```python
from build123d import *

# Parameters (mm, degrees)
SKETCH1_W           = 150
SKETCH1_H           = 150
BOSS_EXTRUDE1_DEPTH = 3
SKETCH2_R           = 2.125
SKETCH2_R_2         = 25
CUT_EXTRUDE3_DEPTH  = 107.108435103
SKETCH3_W           = 10
SKETCH3_H           = 74
SKETCH3_R           = 2.125
BOSS_EXTRUDE2_DEPTH = 3
BOSS_EXTRUDE3_DEPTH = 3


with BuildPart() as part:
    # Sketch1 → Boss-Extrude1 (new body)
    with BuildSketch(Plane(origin=(0, 0, 0), x_dir=(1, 0, 0), z_dir=(0, 1, 0))):
        Rectangle(SKETCH1_W, SKETCH1_H)
    extrude(amount=BOSS_EXTRUDE1_DEPTH)

    # Sketch2 → Cut-Extrude3 (cut, through all)
    with BuildSketch(Plane(origin=(0, 3, 0), x_dir=(1, 0, 0), z_dir=(0, 1, 0))):
        with Locations(Location((-65, -44.8, 0), (0, 0, 270))):
            Circle(SKETCH2_R)
        with Locations(Location((-65, 44.8, 0), (0, 0, 90))):
            Circle(SKETCH2_R)
        with Locations(Location((-44.8, 65, 0), (0, 0, 270))):
            Circle(SKETCH2_R)
        with Locations(Location((44.8, 65, 0), (0, 0, 90))):
            Circle(SKETCH2_R)
        with Locations(Location((65, 44.8, 0), (0, 0, 270))):
            Circle(SKETCH2_R)
        with Locations(Location((65, -44.8, 0), (0, 0, 90))):
            Circle(SKETCH2_R)
        with Locations(Location((44.8, -65, 0), (0, 0, 270))):
            Circle(SKETCH2_R)
        with Locations(Location((-44.8, -65, 0), (0, 0, 90))):
            Circle(SKETCH2_R)
        with Locations(Location((0, 0, 0), (0, 0, 270))):
            Circle(SKETCH2_R_2)
    extrude(amount=-CUT_EXTRUDE3_DEPTH, mode=Mode.SUBTRACT)

    # Sketch3 → Boss-Extrude2 (add)
    # profile 1 of 2: a face of its own
    with BuildSketch(Plane(origin=(0, 3, 0), x_dir=(1, 0, 0), z_dir=(0, 1, 0))):
        with Locations((-80, 0)):
            Rectangle(SKETCH3_W, SKETCH3_H)
        with Locations(Location((-80, 32, 0), (0, 0, 270))):
            Circle(SKETCH3_R, mode=Mode.SUBTRACT)
        with Locations(Location((-80, -32, 0), (0, 0, 90))):
            Circle(SKETCH3_R, mode=Mode.SUBTRACT)
    # profile 2 of 2: a face of its own
    with BuildSketch(Plane(origin=(0, 3, 0), x_dir=(1, 0, 0), z_dir=(0, 1, 0))):
        with Locations((80, 0)):
            Rectangle(SKETCH3_W, SKETCH3_H)
        with Locations(Location((80, -32, 0), (0, 0, 270))):
            Circle(SKETCH3_R, mode=Mode.SUBTRACT)
        with Locations(Location((80, 32, 0), (0, 0, 90))):
            Circle(SKETCH3_R, mode=Mode.SUBTRACT)
    extrude(amount=-BOSS_EXTRUDE2_DEPTH)

    # Sketch4 → Boss-Extrude3 (add)
    with BuildSketch(Plane(origin=(0, 3, 0), x_dir=(1, 0, 0), z_dir=(0, 1, 0))):
        Polygon((-85, 37), (-75, 47), (-75, 37), align=None)
        Polygon((75, 47), (75, 37), (85, 37), align=None)
        Polygon((85, -37), (75, -47), (75, -37), align=None)
        Polygon((-75, -47), (-75, -37), (-85, -37), align=None)
    extrude(amount=-BOSS_EXTRUDE3_DEPTH)


solid = part.part
```
Can you work these out from the model? Positions are in its coordinate system, mm. Round coordinates to 2 decimals unless told otherwise and drop trailing zeros. Order: outer loops, then holes, each group sorted by start corner. A loop starts at its lowest first (then second) coordinate and runs counter-clockwise, first axis right, second up.
(1) I'm going to push a flat-ended pin straight in: pin 1 (0.9 mm diameter, centred on y = 1, z = -65, fed in from -X). Where does the tip first touch, or does it pass through?
Results are:
pin 1: stops at x = -75
(2) If we section it at D-D (z = -65): Please give me the cut outline in (x, y) (3 decimals).
Results are:
outline: (-75, 0) - (-46.925, 0) - (-46.925, 3) - (-75, 3) - close; (-42.675, 0) - (42.675, 0) - (42.675, 3) - (-42.675, 3) - close; (46.925, 0) - (75, 0) - (75, 3) - (46.925, 3) - close
(3) If we section it at A-A (z = 0): Please give me the cut outline in (x, y), plus the area to 3 significant figures.
Results are:
outline: (-85, 0) - (-25, 0) - (-25, 3) - (-85, 3) - close; (25, 0) - (85, 0) - (85, 3) - (25, 3) - close
area: 360 mm2
(4) We'd pull the mould along Z, two halves only. Please class faces 1 (the face through (-80, 2, 42)), 2 (the face through (44.707, 1.521, -62.877)), 3 (the face through (-82.107, 1.521, 32.277)), 4 (the face through (-18, 0, -18)): +Z half, -Z half, draft (parallel to the pull), parting line (faces both ways), or undercut.
Results are:
face 1: +Z half
face 2: undercut
face 3: undercut
face 4: draft
(5) If we section it at B-B (y = 1.65): Count the separate pieces of the cut face and the enclosed holes in it, plus the area to 3 significant figures.
Results are:
separate pieces: 1
enclosed holes: 13
area: 22,000 mm2
(6) If we section it at C-C (x = 0): Please give me the cut outline in (y, z), plus the area to 3 significant figures.
Results are:
outline: (0, -75) - (3, -75) - (3, -25) - (0, -25) - close; (0, 25) - (3, 25) - (3, 75) - (0, 75) - close
area: 300 mm2
(7) If I drill on L1, parallel to X at y = 1.85, z = 65 (3 decimals); L2, parallel to Z at x = -43.5, y = 2.1; L3, parallel to X at y = 2.05, z = -44.8 (3 decimals), over which ranges is the centre line in solid material (lowest first)?
Results are:
L1: x = -75 to -46.925, -42.675 to 42.675, 46.925 to 75
L2: z = -75 to -66.68, -63.32 to 63.32, 66.68 to 75
L3: x = -77.2 to -67.125, -62.875 to 62.875, 67.125 to 77.2
